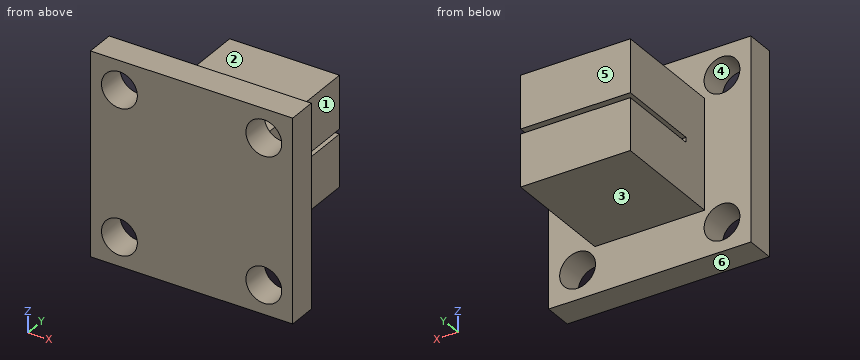
from build123d import *

# Parameters (mm, degrees)
F0_W     = 35
F0_H     = 35
F1_DEPTH = 5
F2_R     = 3.1
F3_DEPTH = 5.001
F4_W     = 19
F4_H     = 19
F5_DEPTH = 20
F6_W     = 19
F6_H     = 0.85
F7_DEPTH = 15


with BuildPart() as f1:
    # F0 (on Front) → F1 (new body)
    with BuildSketch(Plane.XZ):
        with Locations((0.559466, -17.5)):
            Rectangle(F0_W, F0_H)
    extrude(amount=F1_DEPTH)

    # F2 (on face) → F3 (cut, through all)
    with BuildSketch(Plane(origin=(0, 0, 0), x_dir=(-1, 0, 0), z_dir=(0, 1, 0))):
        with Locations((-13.059466, -5)):
            Circle(F2_R)
        with Locations((11.940534, -5)):
            Circle(F2_R)
        with Locations((-13.059466, -30)):
            Circle(F2_R)
        with Locations((11.940534, -30)):
            Circle(F2_R)
    extrude(amount=-F3_DEPTH, mode=Mode.SUBTRACT)

    # F4 (on face) → F5 (join)
    with BuildSketch(Plane(origin=(0, 0, 0), x_dir=(-1, 0, 0), z_dir=(0, 1, 0))):
        with Locations((-0.559466, -17.5)):
            Rectangle(F4_W, F4_H)
    extrude(amount=F5_DEPTH)

    # F6 (on face) → F7 (cut)
    with BuildSketch(Plane(origin=(0, 20, 0), x_dir=(-1, 0, 0), z_dir=(0, 1, 0))):
        with Locations((-0.559466, -17.575)):
            Rectangle(F6_W, F6_H)
    extrude(amount=-F7_DEPTH, mode=Mode.SUBTRACT)


solid = f1.part
CAD build for the part. Positions are in the model's coordinates, mm. Face numbers are marked on the shaded views. A direction names the side the tool comes from. Coordinates: 2 decimals unless noted, no trailing zeros. Write each loop counter-clockwise with the first axis right and the second up, starting at its lowest first coordinate (ties: lowest second). Pieces come first, ordered by that corner, then holes. Notation, with made-up numbers: M -31.75,-29 L 10.25,-29 A21 ccw 10.25,-19 Z; hole C 82,23 d4. An arc over 180 degrees is marked long. Return JSON: item names as keys, results as strings.
Item 1: Probe line 1 (Z direction, x = 15, y = -1); line 2 (Z direction, x = -10.5, y = -4); line 3 (Y direction, x = 5, z = -33). List the from-to ranges inside material, lowest first. Write a range as from..to.
Findings below:
{"line 1": "z = -35..-32.42, -27.58..-7.42, -2.58..0", "line 2": "z = -35..-32.74, -27.26..-7.74, -2.26..0", "line 3": "y = -5..0"}
Item 2: Slice it at A-A, the plane z = -30. Write the cut outline in (x, y), and give its area (3 significant figures).
Findings below:
{"outline": "M -16.94,-5 L -15.04,-5 L -15.04,0 L -16.94,0 Z; M -8.84,-5 L 9.96,-5 L 9.96,0 L -8.84,0 Z; M 16.16,-5 L 18.06,-5 L 18.06,0 L 16.16,0 Z", "area": "113 mm2"}
Item 3: Slice it at C-C, the plane x = -12. Write the cut outline in (y, z), and give its area (3 significant figures).
Findings below:
{"outline": "M -5,-35 L 0,-35 L 0,-33.1 L -5,-33.1 Z; M -5,-26.9 L 0,-26.9 L 0,-8.1 L -5,-8.1 Z; M -5,-1.9 L 0,-1.9 L 0,0 L -5,0 Z", "area": "113 mm2"}
Item 4: Slice it at B-B, the plane y = 15. Write the cut outline in (x, z).
Findings below:
{"outline": "M -8.94,-27 L 10.06,-27 L 10.06,-18 L -8.94,-18 Z; M -8.94,-17.15 L 10.06,-17.15 L 10.06,-8 L -8.94,-8 Z"}
Item 5: Slice it at D-D, the plane z = -18.5. Write the cut outline in (x, y), and give its area (3 significant figures).
Findings below:
{"outline": "M -16.94,-5 L 18.06,-5 L 18.06,0 L 10.06,0 L 10.06,20 L -8.94,20 L -8.94,0 L -16.94,0 Z", "area": "555 mm2"}
Item 6: Two-plate mould, pull along Z, no slides. Class the marked faces 4, 5 and 6: +Z half, -Z half, draft (parallel to the pull), parting line (faces both ways), or undercut.
Findings below:
{"face 4": "undercut", "face 5": "draft", "face 6": "-Z half"}
Item 7: Which spindle directions (+Z, -Z, +X, -X, +Y, -Y) get a long thin tool onto all of the face, cutting with end or side? Do the marked faces 1, 2 and 3. Say none if no direction does.
Findings below:
{"face 1": "+Z, -Z, +X, +Y", "face 2": "+Z, +X, -X, +Y", "face 3": "-Z, +X, -X, +Y"}
Item 8: Drop flat-ended pins along their axis: pin 1 Ø8 at (x, z) = (13.06, -5) entering from +Y; pin 2 Ø5.5 at (x, y) = (0.5, 12.5) entering from +Z; pin 3 Ø6 at (x, y) = (2.5, 15.5) entering from -Z. Give the stop position or say it passes through.
Findings below:
{"pin 1": "stops at y = 0", "pin 2": "stops at z = -8", "pin 3": "stops at z = -27"}
